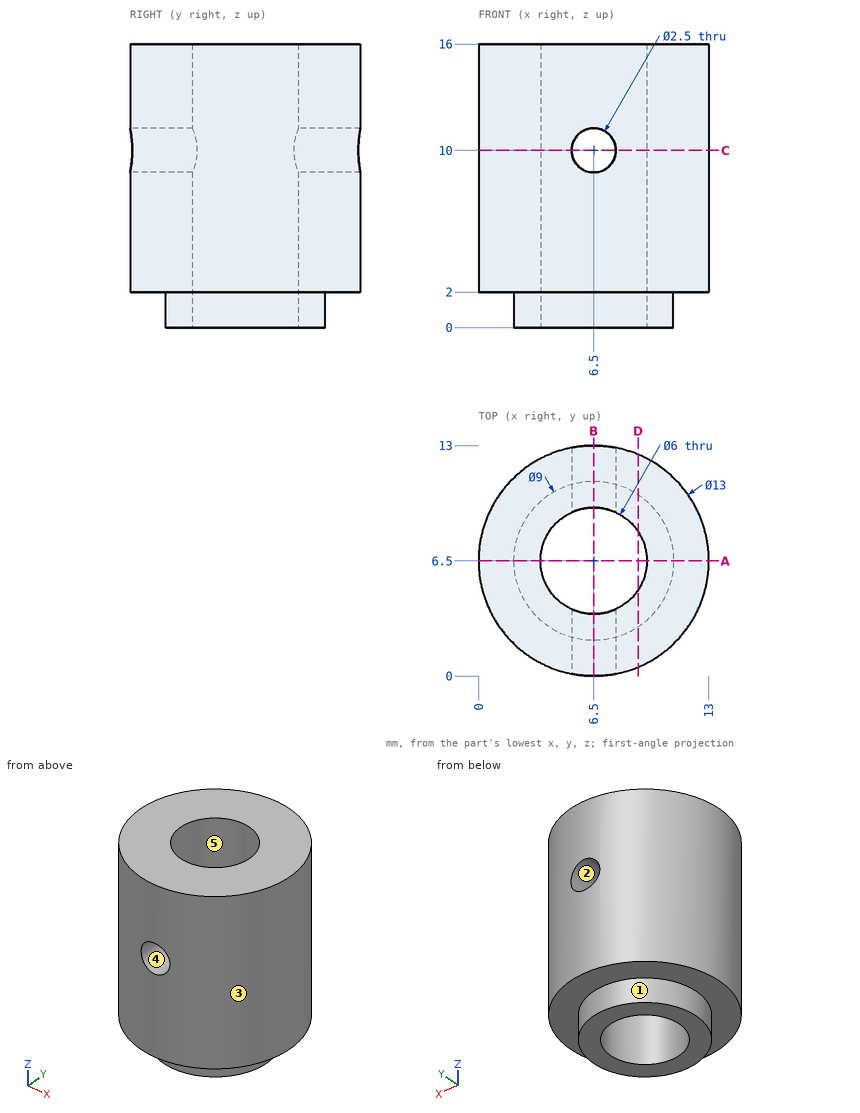
For this review, use the dimensioned drawing (mm, ordinates from the lowest corner) and the shaded views. A direction names the side the tool comes from. Give positions to 0.01 mm unless a question says otherwise; leave off trailing zeros. Order: outer loops, then holes, each group sorted by start corner. A loop starts at its lowest first (then second) coordinate and runs counter-clockwise, first axis right, second up.
1) The part is to be moulded in two halves that separate along Y. For the marked faces 3, 4 and 5, say which applies: released by +Y, released by -Y, zero draft, split by the parting line, or undercut.
2) For the marked faces 1 and 2, list the 3-axis set-ups (+Z, -Z, +X, -X, +Y, -Y) from which the entire face can be reached by the end or side of a thin tool; tool diameter is ignored.
3) Insertion check: pin 1 (1.5 mm diameter, centred on x = 5.5, y = 6, fed in from -Z); pin 2 (1.5 mm diameter, centred on x = 1.5, y = 10, fed in from -Z); pin 3 (1 mm diameter, centred on y = 10, z = 9, fed in from -X). Each pin has a flat end and moves straight along its axis. Give the tip position at first contact, or say it passes through.
4) Wall thickness on line 1 (Z direction, x = 1, y = 4.5); line 2 (Y direction, x = 4.75, z = 1.5); line 3 (X direction, y = 6.75, z = 15): over which ranges is each line inside the solid? List them lowest first.
5) Take a section at B-B (x = 6.5). Give the boundary of the cut face in (y, z).
6) Take a section at A-A (y = 6.5). Give the boundary of the cut face in (x, z), then the cut area to 3 significant figures.
7) Take a section at D-D (x = 9). Give the boundary of the cut face in (y, z).
8) Take a section at C-C (z = 10). Give the boundary of the cut face in (x, y), then the cut area to 3 significant figures.
Derived:
1. face 3: split by the parting line
1. face 4: zero draft
1. face 5: undercut
2. face 1: -Z
2. face 2: +Y, -Y
3. pin 1: passes through
3. pin 2: stops at z = 2
3. pin 3: stops at x = 0.73
4. line 1: z = 2 to 16
4. line 2: y = 2.35 to 4.06, 8.94 to 10.65
4. line 3: x = 0 to 3.51, 9.49 to 13
5. outline: (0, 2) - (2, 2) - (2, 0) - (3.5, 0) - (3.5, 8.75) - (0, 8.75) - close; (0, 11.25) - (3.5, 11.25) - (3.5, 16) - (0, 16) - close; (9.5, 0) - (11, 0) - (11, 2) - (13, 2) - (13, 8.75) - (9.5, 8.75) - close; (9.5, 11.25) - (13, 11.25) - (13, 16) - (9.5, 16) - close
6. outline: (0, 2) - (2, 2) - (2, 0) - (3.5, 0) - (3.5, 16) - (0, 16) - close; (9.5, 0) - (11, 0) - (11, 2) - (13, 2) - (13, 16) - (9.5, 16) - close
6. area: 104 mm2
7. outline: (0.5, 2) - (2.76, 2) - (2.76, 0) - (4.84, 0) - (4.84, 16) - (0.5, 16) - close; (8.16, 0) - (10.24, 0) - (10.24, 2) - (12.5, 2) - (12.5, 16) - (8.16, 16) - close
8. outline: (5.25, 0.12) - (5.25, 3.77) arc R3 cw to (5.25, 9.23) - (5.25, 12.88) arc R6.5 ccw to start; (7.75, 0.12) arc R6.5 ccw to (7.75, 12.88) - (7.75, 9.23) arc R3 cw to (7.75, 3.77) - close
8. area: 86.7 mm2
